Could you check a few things on this model? Use its own coordinates, in mm. Face numbers are marked on the shaded views. Coordinates: 2 decimals unless noted, no trailing zeros. Loops run counter-clockwise (first coordinate to the right, second up) from the corner with the lowest first, then second, coordinate; pieces in that order, holes last. Notation, with made-up numbers: (44, -31) -> (66, -31) arc R19 ccw to (66, -1) -> close; hole circle Ø6 at (17, -29). An arc over 180 degrees is marked (long way). One line per question, with ' | ' between items.
```python
from build123d import *

# Parameters (mm, degrees)
BOSS_EXTRUDE1_DEPTH = 0.5
BOSS_EXTRUDE2_DEPTH = 1.2
SKETCH3_W           = 8
SKETCH3_H           = 2
CUT_EXTRUDE1_DEPTH  = 1
BOSS_EXTRUDE3_DEPTH = 1
FILLET1_R           = 3
SKETCH5_R           = 1.6
CUT_EXTRUDE2_DEPTH  = 1


with BuildPart() as part:
    # Sketch1 → Boss-Extrude1 (new body)
    with BuildSketch(Plane(origin=(0, 0, 0), x_dir=(1, 0, 0), z_dir=(0, 1, 0))):
        with BuildLine():
            Line((-20.743902439, 24.603658537), (27.756097561, 24.603658537))
            Line((27.756097561, 24.603658537), (27.756097561, -23.896341463))
            Line((27.756097561, -23.896341463), (12.506097561, -23.896341463))
            ThreePointArc((12.506097561, -23.896341463), (10.384777217, -24.77502112), (9.506097561, -26.896341463))
            Line((9.506097561, -26.896341463), (9.506097561, -68.896341463))
            Line((9.506097561, -68.896341463), (-2.493902439, -68.896341463))
            Line((-2.493902439, -68.896341463), (-2.493902439, -26.896341463))
            ThreePointArc((-2.493902439, -26.896341463), (-3.372582095, -24.77502112), (-5.493902439, -23.896341463))
            Line((-5.493902439, -23.896341463), (-20.743902439, -23.896341463))
            Line((-20.743902439, -23.896341463), (-20.743902439, 24.603658537))
        make_face()
        with BuildLine():
            Line((-18.743902439, 22.603658537), (25.756097561, 22.603658537))
            Line((25.756097561, 22.603658537), (25.756097561, -21.896341463))
            Line((25.756097561, -21.896341463), (12.506097561, -21.896341463))
            ThreePointArc((12.506097561, -21.896341463), (8.970563655, -23.360807557), (7.506097561, -26.896341463))
            Line((7.506097561, -26.896341463), (7.506097561, -66.896341463))
            Line((7.506097561, -66.896341463), (-0.493902439, -66.896341463))
            Line((-0.493902439, -66.896341463), (-0.493902439, -26.896341463))
            ThreePointArc((-0.493902439, -26.896341463), (-1.958368533, -23.360807557), (-5.493902439, -21.896341463))
            Line((-5.493902439, -21.896341463), (-18.743902439, -21.896341463))
            Line((-18.743902439, -21.896341463), (-18.743902439, 22.603658537))
        make_face(mode=Mode.SUBTRACT)
    extrude(amount=BOSS_EXTRUDE1_DEPTH)

    # Sketch2 → Boss-Extrude2 (add)
    with BuildSketch(Plane(origin=(0, 0.5, 0), x_dir=(1, 0, 0), z_dir=(0, 1, 0))):
        with BuildLine():
            Line((-20.743902439, 24.603658537), (-20.743902439, -23.896341463))
            Line((-20.743902439, -23.896341463), (-5.493902439, -23.896341463))
            ThreePointArc((-5.493902439, -23.896341463), (-3.372582095, -24.77502112), (-2.493902439, -26.896341463))
            Line((-2.493902439, -26.896341463), (-2.493902439, -68.896341463))
            Line((-2.493902439, -68.896341463), (9.506097561, -68.896341463))
            Line((9.506097561, -68.896341463), (9.506097561, -26.896341463))
            ThreePointArc((9.506097561, -26.896341463), (10.384777217, -24.77502112), (12.506097561, -23.896341463))
            Line((12.506097561, -23.896341463), (27.756097561, -23.896341463))
            Line((27.756097561, -23.896341463), (27.756097561, 24.603658537))
            Line((27.756097561, 24.603658537), (-20.743902439, 24.603658537))
        make_face()
    extrude(amount=BOSS_EXTRUDE2_DEPTH)

    # Sketch3 → Cut-Extrude1 (cut)
    with BuildSketch(Plane.XZ):
        with Locations((3.506097561, 67.896341463)):
            Rectangle(SKETCH3_W, SKETCH3_H)
    extrude(amount=-CUT_EXTRUDE1_DEPTH, mode=Mode.SUBTRACT)

    # Sketch4 → Boss-Extrude3 (add)
    with BuildSketch(Plane(origin=(0, 1.7, 0), x_dir=(1, 0, 0), z_dir=(0, 1, 0))):
        Polygon((-12.493902439, -33.896341463), (19.506097561, -33.896341463), (37.756097561, -33.896341463), (37.756097561, 34.603658537), (-30.743902439, 34.603658537), (-30.743902439, -33.896341463), align=None)
    extrude(amount=-BOSS_EXTRUDE3_DEPTH)

    # Fillet1
    fillet1_edges = [part.edges().sort_by_distance(p)[0] for p in [
        (37.756097561, 1.2, 33.896341463),
        (37.756097561, 1.2, -34.603658537),
        (-30.743902439, 1.2, 33.896341463),
        (-30.743902439, 1.2, -34.603658537),
    ]]
    fillet(fillet1_edges, radius=FILLET1_R)

    # Sketch5 → Cut-Extrude2 (cut)
    with BuildSketch(Plane.XZ.offset(-0.7)):
        with Locations(Location((-24.743902439, 27.896341463, 0), (0, 0, 270))):  # turned: the seam where the file's is
            Circle(SKETCH5_R)
        with Locations(Location((31.756097561, 27.896341463, 0), (0, 0, 270))):  # turned: the seam where the file's is
            Circle(SKETCH5_R)
        with Locations(Location((31.756097561, -28.603658537, 0), (0, 0, 270))):  # turned: the seam where the file's is
            Circle(SKETCH5_R)
        with Locations(Location((-24.743902439, -28.603658537, 0), (0, 0, 270))):  # turned: the seam where the file's is
            Circle(SKETCH5_R)
    extrude(amount=-CUT_EXTRUDE2_DEPTH, mode=Mode.SUBTRACT)


solid = part.part
```
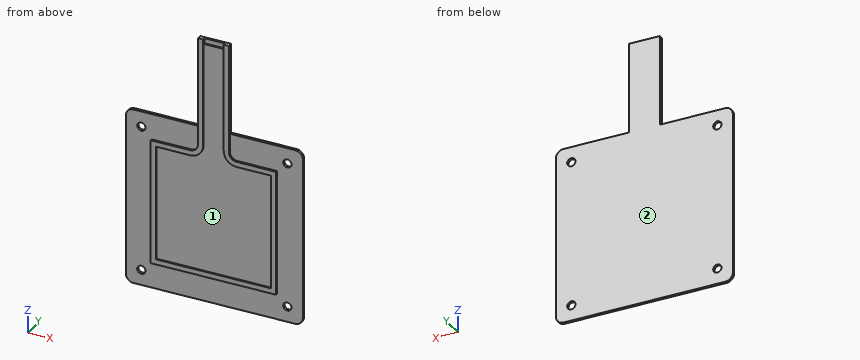
Q1. We'd pull the mould along X, two halves only. Please class the marked faces 1 and 2: released by +X, released by -X, zero draft, split by the parting line, or undercut.
Values follow:
face 1: undercut | face 2: zero draft
Q2. Please list where these lines run through material, in increasing order: L1, parallel to X at y = 0.2, z = 48; L2, parallel to X at y = 0.25, z = -14; L3, parallel to Z at x = -26, y = 1.55. Write a range as [from, to].
Values follow:
L1: x = [-2.49, -0.49], [7.51, 9.51] | L2: x = [-20.74, -18.74], [25.76, 27.76] | L3: z = [-34.6, -29.59], [-27.61, 26.91], [28.89, 33.9]
Q3. Imagine slicing it at C-C on z = -9. Write out the boundary of the cut face in (x, y).
Values follow:
outline: (-30.74, 0.7) -> (-20.74, 0.7) -> (-20.74, 0) -> (-18.74, 0) -> (-18.74, 0.5) -> (25.76, 0.5) -> (25.76, 0) -> (27.76, 0) -> (27.76, 0.7) -> (37.76, 0.7) -> (37.76, 1.7) -> (-30.74, 1.7) -> close
Q4. For pin 1 (1.6 mm diameter, centred on x = 5, z = 67.5, fed in from -Y); pin 2 (1 mm diameter, centred on x = -18.5, y = 1, fed in from +Z); pin 3 (0.8 mm diameter, centred on y = 0.5, z = 45.5, fed in from -X), each with a flat end and sliding along its axis, tell me the tip position at first contact or that it passes through.
Values follow:
pin 1: stops at y = 0.5 | pin 2: stops at z = 33.9 | pin 3: stops at x = -2.49
Q5. Imagine slicing it at B-B on x = 3. Write out the boundary of the cut face in (y, z), plus the area to 3 significant figures.
Values follow:
outline: (0, -24.6) -> (0.7, -24.6) -> (0.7, -34.6) -> (1.7, -34.6) -> (1.7, 68.9) -> (1, 68.9) -> (1, 66.9) -> (0.5, 66.9) -> (0.5, -22.6) -> (0, -22.6) -> close | area: 122 mm2
Q6. Imagine slicing it at A-A on z = 28.5. Write out the boundary of the cut face in (x, y), plus the area to 3 significant figures.
Values follow:
outline: (-30.74, 0.7) -> (-26.23, 0.7) -> (-26.23, 1.7) -> (-30.74, 1.7) -> close; (-23.26, 0.7) -> (-2.49, 0.7) -> (-2.49, 0) -> (-0.49, 0) -> (-0.49, 0.5) -> (7.51, 0.5) -> (7.51, 0) -> (9.51, 0) -> (9.51, 0.7) -> (30.27, 0.7) -> (30.27, 1.7) -> (-23.26, 1.7) -> close; (33.24, 0.7) -> (37.76, 0.7) -> (37.76, 1.7) -> (33.24, 1.7) -> close | area: 67.0 mm2
Q7. Imagine slicing it at D-D on y = 1.3. Write out the boundary of the cut face in (x, z).
Values follow:
outline: (-30.74, -31.6) arc R3 ccw to (-27.74, -34.6) -> (34.76, -34.6) arc R3 ccw to (37.76, -31.6) -> (37.76, 30.9) arc R3 ccw to (34.76, 33.9) -> (9.51, 33.9) -> (9.51, 68.9) -> (-2.49, 68.9) -> (-2.49, 33.9) -> (-27.74, 33.9) arc R3 ccw to (-30.74, 30.9) -> close; hole circle Ø3.2 at (-24.74, -28.6); hole circle Ø3.2 at (-24.74, 27.9); hole circle Ø3.2 at (31.76, -28.6); hole circle Ø3.2 at (31.76, 27.9)
